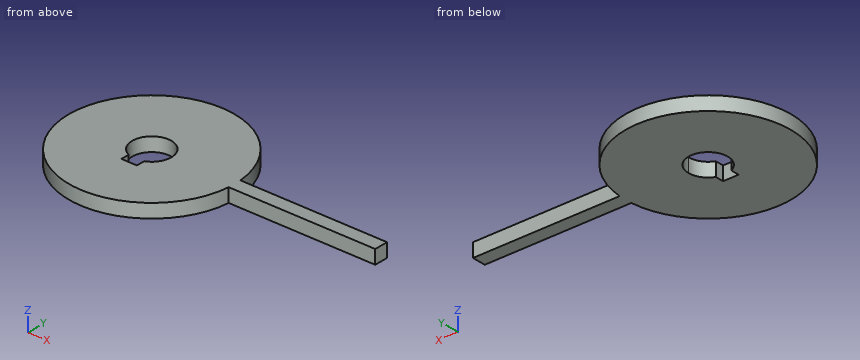
from build123d import *

# Parameters (mm, degrees)
F1_DEPTH = 5


with BuildPart() as f1:
    # F0 (on Top) → F1 (new body)
    with BuildSketch(Plane.XY):
        with BuildLine():
            ThreePointArc((29.892959, -2.5), (29.96573, -1.295459), (29.99, -0.088966))
            ThreePointArc((29.99, -0.088966), (29.962007, 1.206726), (29.878079, 2.5))
            ThreePointArc((29.878079, 2.5), (-30.009867, -0.178242), (29.892959, -2.5))
        make_face()
        with BuildLine():
            ThreePointArc((-2.81, -6.613535), (-3.917044, 5.839356), (7.09, -0.088966))
            ThreePointArc((7.09, -0.088966), (5.918322, -3.996011), (2.79, -6.613535))
            Line((2.79, -6.613535), (2.79, -9.688966))
            Line((2.79, -9.688966), (-0.01, -9.688966))
            Line((-0.01, -9.688966), (-2.81, -9.688966))
            Line((-2.81, -9.688966), (-2.81, -6.613535))
        make_face(mode=Mode.SUBTRACT)
        with BuildLine():
            ThreePointArc((29.878079, 2.5), (29.962007, 1.206726), (29.99, -0.088966))
            ThreePointArc((29.99, -0.088966), (29.96573, -1.295459), (29.892959, -2.5))
            Line((29.892959, -2.5), (82.989869, -2.5))
            Line((82.989869, -2.5), (82.989869, 0))
            Line((82.989869, 0), (82.989869, 2.5))
            Line((82.989869, 2.5), (29.878079, 2.5))
        make_face()
    extrude(amount=F1_DEPTH)


solid = f1.part
Check sheet for the modelled part. Datum: model origin and axes. Units: mm. Give positions to 0.01 mm unless a question says otherwise; leave off trailing zeros. Write each loop counter-clockwise with the first axis right and the second up, starting at its lowest first coordinate (ties: lowest second). Pieces come first, ordered by that corner, then holes. Notation, with made-up numbers: M 76.25,74.25 L 115.25,74.25 A14 cw 115.25,96.25 Z; hole C 13.5,13 d6. An arc over 180 degrees is marked long. Use one line per item in the form item = value.
(1) Depth check by flat-ended pin: P1, Ø1.5, axis at x = 13, z = 3.5, coming from the -Y side; P2, Ø3, axis at x = 65.5, z = 4, coming from the +Y side; P3, Ø0.9, axis at y = -9, z = 2, coming from the +X side; P4, Ø13, axis at x = -0.01, y = -0.09, coming from the +Z side. Enter the tip coordinate at first touch or a pass-through.
Answer block:
P1 = -27.47
P2 = 2.5
P3 = 28.77
P4 = through
(2) Section check D-D on x = 47.5. Record the boundary of the cut face in (y, z), plus the area to 3 significant figures.
Answer block:
outline = M -2.5,0 L 2.5,0 L 2.5,5 L -2.5,5 Z
area = 25.0 mm2
(3) Section check C-C on y = -5. Record the boundary of the cut face in (x, z), plus the area to 3 significant figures.
Answer block:
outline = M -29.61,0 L -5.14,0 L -5.14,5 L -29.61,5 Z; M 5.12,0 L 29.59,0 L 29.59,5 L 5.12,5 Z
area = 245 mm2
(4) Material ranges on line 1 along Y through (x, z) = (-0.01, 1.25); line 2 along X through (y, z) = (0, 4); line 3 along Y through (x, z) = (62.5, 2.1), recorded low to high.
Answer block:
line_1 = -30.09 to -9.69, 7.01 to 29.91
line_2 = -30.01 to -7.11, 7.09 to 82.99
line_3 = -2.5 to 2.5
(5) Section check A-A on x = -0.01. Record the boundary of the cut face in (y, z).
Answer block:
outline = M -30.09,0 L -9.69,0 L -9.69,5 L -30.09,5 Z; M 7.01,0 L 29.91,0 L 29.91,5 L 7.01,5 Z
(6) Section check B-B on z = 3.55. Record the boundary of the cut face in (x, y), plus the area to 3 significant figures.
Answer block:
outline = M 29.88,2.5 A30 ccw long 29.89,-2.5 L 82.99,-2.5 L 82.99,2.5 Z; hole M -2.81,-9.69 L 2.79,-9.69 L 2.79,-6.61 A7.1 ccw long -2.81,-6.61 Z
area = 2,920 mm2
